Verification items for the finished model (mm, model axes). Coordinates: 2 decimals unless noted, no trailing zeros. Order: outer loops, then holes, each group sorted by start corner. A loop starts at its lowest first (then second) coordinate and runs counter-clockwise, first axis right, second up. Notation, with made-up numbers: M 89.25,76 L 144.25,76 A23 ccw 144.25,112 Z; hole C 26.25,76.25 d4. An arc over 180 degrees is marked long. Return JSON: item names as keys, results as strings.
```python
from build123d import *

# Parameters (mm, degrees)
F0_R     = 10
F1_DEPTH = 200
F4_D     = 3
F4_DEPTH = 100
F6_D     = 15
F6_DEPTH = 200


with BuildPart() as f1:
    # F0 (on Top) → F1 (new body)
    with BuildSketch(Plane.XY):
        Circle(F0_R)
    extrude(amount=F1_DEPTH)

    # F4
    with Locations(Plane(origin=(0, 0, 0), x_dir=(1, 0, 0), z_dir=(0, 0, -1))):
        with Locations((0, 0)):
            Hole(F4_D / 2, depth=F4_DEPTH)

    # F6
    with Locations(Plane.XY.offset(200)):
        with Locations((0, 0)):
            Hole(F6_D / 2, depth=F6_DEPTH)


solid = f1.part
```
Q1. Draft check along X on faces 1 (the face through (-2.17, -9.76, 98.6)), 2 (the face through (4, 7, 200)), 3 (the face through (7.493, 0.33, 98.6)). Enter one of: pulls with the +X half, pulls with the -X half, needs draft (parallel to the pull), parting line crosses it, or undercut.
Values:
{"face 1": "parting line crosses it", "face 2": "needs draft", "face 3": "undercut"}
Q2. Cross-section at C-C, the plane z = 45. Record the boundary of the cut face in (x, y).
Values:
{"outline": "C 0,0 d20; hole C 0,0 d15"}
Q3. Cross-section at A-A, the plane y = 0. Record the boundary of the cut face in (x, z), and give its area (3 significant figures).
Values:
{"outline": "M -10,0 L -7.5,0 L -7.5,200 L -10,200 Z; M 7.5,0 L 10,0 L 10,200 L 7.5,200 Z", "area": "1,000 mm^2"}
Q4. Material ranges on line 1 along Y through (x, z) = (0, 140); line 2 along X through (y, z) = (-1, 178); line 3 along Y through (x, z) = (-5, 55), recorded low to high.
Values:
{"line 1": "-10 to -7.5, 7.5 to 10", "line 2": "-9.95 to -7.43, 7.43 to 9.95", "line 3": "-8.66 to -5.59, 5.59 to 8.66"}
Q5. Go/stop test with flat-tipped pins: pin 1 (6 mm diameter, centred on y = -6, z = 53, fed in from -X); pin 2 (3 mm diameter, centred on x = 5.5, z = 179.5, fed in from +Y); pin 3 (4 mm diameter, centred on x = 1, y = -6, fed in from -Z); pin 4 (1.5 mm diameter, centred on x = 3.5, z = 57, fed in from -Y). Record where each tip stops, or that it passes through.
Values:
{"pin 1": "x = -9.54", "pin 2": "y = 9.17", "pin 3": "z = 0", "pin 4": "y = -9.61"}
